Read the model definition and answer for the solid it produces. Units are mm, in the model's axes. Give positions to 0.01 mm unless a question says otherwise; leave off trailing zeros. Order: outer loops, then holes, each group sorted by start corner. A loop starts at its lowest first (then second) coordinate and runs counter-clockwise, first axis right, second up. Notation, with made-up numbers: (16, -16) -> (54, -16) arc R19 cw to (54, 2) -> close; hole circle Ø11 at (14, -37). An arc over 180 degrees is marked (long way). One line per question, with ' | ' between items. Start each with the question number.
Autodesk Inventor part; units mm, degrees
ref_plane "YZ Plane" through (0, 0, 0) normal (1, 0, 0) x (0, 1, 0)
ref_plane "XZ Plane" through (0, 0, 0) normal (0, 1, 0) x (-1, 0, 0)
ref_plane "XY Plane" through (0, 0, 0) normal (0, 0, 1) x (1, 0, 0)
sketch "Sketch1" plane through (0, 0, 0) normal (0, 0, 1) x (1, 0, 0)
  line L0 (0, 0) -> (25, 0)
  line L1 (25, 0) -> (25, 25)
  line L2 (25, 25) -> (0, 25)
  line L3 (0, 25) -> (0, 0)
  line L4 (23.5, 23.5) -> (23.5, 1.5)
  line L5 (23.5, 1.5) -> (1.5, 1.5)
  line L6 (1.5, 1.5) -> (1.5, 23.5)
  line L7 (1.5, 23.5) -> (23.5, 23.5)
  dimension "d0" = 25
  dimension "d1" = 25
  dimension "d2" = 1.5
extrude "Extrusion1" add sketch "Sketch1" along normal blind 850
sketch "Sketch2" plane through (0, 0, 0) normal (1, 0, 0) x (0, 0, -1)
  line L0 (0, 0) -> (0, 25)
  line L1 (-850, 0) -> (-850, 25)
  point P0 (-837.5, 12.5)
  point P1 (-12.5, 12.5)
  dimension "d5" = 12.5
  dimension "d6" = 12.5
  dimension "d7" = 12.5
hole "Hole1" at (0, 12.5, 837.5) at (0, 12.5, 12.5) direction (1, 0, 0) diameter 6 end through all counterbore diameter 11 counterbore depth 5
properties part number "Side Bar"
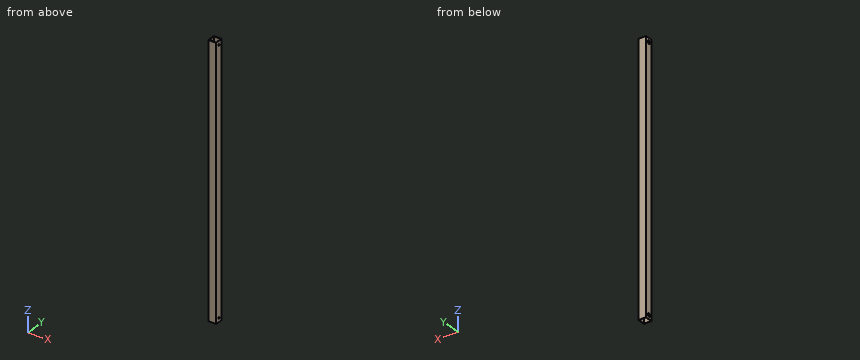
Q1. Given P1, Ø6.5, axis at y = 12.5, z = 12.5, coming from the +X side; P2, Ø9, axis at y = 12.5, z = 837.5, coming from the -X side, each flat-ended and moving along its own axis, determine where each tip first touches the part or whether it passes through.
Q2. Find the intervals of material crossed by line 1 (Z direction, x = 24, y = 12.5); line 2 (Z direction, x = 0.4, y = 12.5); line 3 (Y direction, x = 11.5, z = 473), in increasing order.
Q3. A cutting plane is placed at A-A, the plane x = 14.5. Determine the outline of the cut face in (y, z).
Q4. A cutting plane is placed at B-B, the plane z = 200.5. Determine the outline of the cut face in (x, y).
Geometry results:
1) P1: x = 25 | P2: x = 23.5
2) line 1: 0 to 9.5, 15.5 to 834.5, 840.5 to 850 | line 2: 0 to 7, 18 to 832, 843 to 850 | line 3: 0 to 1.5, 23.5 to 25
3) outline: (0, 0) -> (1.5, 0) -> (1.5, 850) -> (0, 850) -> close; (23.5, 0) -> (25, 0) -> (25, 850) -> (23.5, 850) -> close
4) outline: (0, 0) -> (25, 0) -> (25, 25) -> (0, 25) -> close; hole (1.5, 1.5) -> (23.5, 1.5) -> (23.5, 23.5) -> (1.5, 23.5) -> close
